```python
from build123d import *

# Parameters (mm, degrees)
F0_R     = 13.234543
F0_R_2   = 14.602605
F0_R_3   = 13.234537
F1_DEPTH = 25.4


with BuildPart() as f1:
    # F0 (on Front) → F1 (new body)
    with BuildSketch(Plane.XZ):
        with BuildLine():
            Line((-68.349093, 22.744557), (-61.190916, 22.744557))
            Line((-61.190916, 22.744557), (-61.190916, -6.35))
            Line((-61.190916, -6.35), (-68.349093, -6.35))
            ThreePointArc((-68.349093, -6.35), (-55.153312, -48.774699), (-13.896282, -65.262306))
            Line((-13.896282, -65.262306), (-13.896282, -58.104129))
            Line((-13.896282, -58.104129), (15.198263, -58.104129))
            Line((15.198263, -58.104129), (15.198263, -65.262306))
            ThreePointArc((15.198263, -65.262306), (54.17365, -49.31931), (68.332028, -9.660764))
            Line((68.332028, -9.660764), (63.915444, -9.660764))
            Line((63.915444, -9.660764), (63.915444, 21.790432))
            Line((63.915444, 21.790432), (71.073621, 21.790432))
            ThreePointArc((71.073621, 21.790432), (50.996785, 53.196906), (15.198263, 63.584965))
            Line((15.198263, 63.584965), (15.198263, 56.226362))
            Line((15.198263, 56.226362), (-14.778182, 56.226362))
            Line((-14.778182, 56.226362), (-14.778182, 63.384548))
            ThreePointArc((-14.778182, 63.384548), (-49.081059, 52.973883), (-68.349093, 22.744557))
        make_face()
        with Locations((-34.410097, -31.443559)):
            Circle(F0_R, mode=Mode.SUBTRACT)
        with Locations((30.93718, -28.903559)):
            Circle(F0_R, mode=Mode.SUBTRACT)
        Circle(F0_R_2, mode=Mode.SUBTRACT)
        with Locations((-31.870097, 32.287352)):
            Circle(F0_R_3, mode=Mode.SUBTRACT)
        with Locations((31.860813, 33.441897)):
            Circle(F0_R, mode=Mode.SUBTRACT)
    extrude(amount=F1_DEPTH)


solid = f1.part
```
Work out the finished part from the listing and answer in its coordinate system (mm). A direction names the side the tool comes from. Give positions to 0.01 mm unless a question says otherwise; leave off trailing zeros. Loops run counter-clockwise (first coordinate to the right, second up) from the corner with the lowest first, then second, coordinate; pieces in that order, holes last. Notation, with made-up numbers: (28.25, 17) -> (39.25, 17) arc R12 cw to (39.25, 33) -> close; hole circle Ø11 at (63.25, 44). An arc over 180 degrees is marked (long way). Put each result on its own line as item: value. Start each with the question number.
Item 1: The part is cut by section C-C (y = -2). Give the vertices of the cut face in (x, z), then the cut area to 3 significant figures.
Item 2: The mould has two halves that part along X. Classify faces 4 (the face through (0, -13, -58.104)), 5 (the face through (-61.191, -13, 8)), 6 (the face through (-65, -13, -6.35)): released by +X, released by -X, zero draft, split by the parting line, or undercut.
Item 3: The part is cut by section B-B (x = -4.5). Give the vertices of the cut face in (y, z).
Item 4: The part is cut by section D-D (z = 26.5). Give the vertices of the cut face in (x, y), then the cut area to 3 significant figures.
Item 5: The part is cut by section A-A (z = 0). Give the vertices of the cut face in (x, y), then the cut area to 3 significant figures.
Item 6: Which of the six approach directions +Z, -Z, +X, -X, +Y, -Y give full straight-line access (tool end or side, diameter ignored) to faces 1 (the face through (67, -13, 21.79)), 2 (the face through (15.198, -13, -62)), 3 (the face through (15.198, -13, 60))?
Item 7: Each of these flat-tipped pins is pushed along its axis until it touches: P1, Ø2, axis at y = -15.5, z = 60, coming from the +X side; P2, Ø10, axis at x = 10.5, y = -21.5, coming from the +Z side; P3, Ø6, axis at y = -18.5, z = -2, coming from the +X side. Where does it stop, or does it pass through?
Item 8: Find the intervals of material crossed by L1, parallel to X at y = -22, z = -0.5; L2, parallel to Z at x = 0, y = -6; L3, parallel to Z at x = -38, y = -3, in increasing order. Write a range as [from, to].
Answers below:
1. outline: (-68.35, -6.35) arc R51.66 ccw to (-13.9, -65.26) -> (-13.9, -58.1) -> (15.2, -58.1) -> (15.2, -65.26) arc R51.66 ccw to (68.33, -9.66) -> (63.92, -9.66) -> (63.92, 21.79) -> (71.07, 21.79) arc R52.94 ccw to (15.2, 63.58) -> (15.2, 56.23) -> (-14.78, 56.23) -> (-14.78, 63.38) arc R51.66 ccw to (-68.35, 22.74) -> (-61.19, 22.74) -> (-61.19, -6.35) -> close; hole circle Ø26.47 at (-34.41, -31.44); hole circle Ø26.47 at (-31.87, 32.29); hole circle Ø29.21 at (0, 0); hole circle Ø26.47 at (30.94, -28.9); hole circle Ø26.47 at (31.86, 33.44)
1. area: 11,900 mm2
2. face 4: undercut
2. face 5: released by -X
2. face 6: zero draft
3. outline: (-25.4, -58.1) -> (0, -58.1) -> (0, -13.89) -> (-25.4, -13.89) -> close; (-25.4, 13.89) -> (0, 13.89) -> (0, 56.23) -> (-25.4, 56.23) -> close
4. outline: (-67.39, -25.4) -> (-43.77, -25.4) -> (-43.77, 0) -> (-67.39, 0) -> close; (-19.97, -25.4) -> (20.59, -25.4) -> (20.59, 0) -> (-19.97, 0) -> close; (43.13, -25.4) -> (69.85, -25.4) -> (69.85, 0) -> (43.13, 0) -> close
4. area: 2,310 mm2
5. outline: (-61.19, -25.4) -> (-14.6, -25.4) -> (-14.6, 0) -> (-61.19, 0) -> close; (14.6, -25.4) -> (63.92, -25.4) -> (63.92, 0) -> (14.6, 0) -> close
5. area: 2,440 mm2
6. face 1: +X, +Y, -Y
6. face 2: -Z, +Y, -Y
6. face 3: +Z, +Y, -Y
7. P1: x = 41.19
7. P2: z = 63.61
7. P3: x = 63.92
8. L1: [-61.19, -14.59], [14.59, 63.92]
8. L2: [-58.1, -14.6], [14.6, 56.23]
8. L3: [-61, -44.18], [-18.71, 20.56], [44.02, 59.39]
